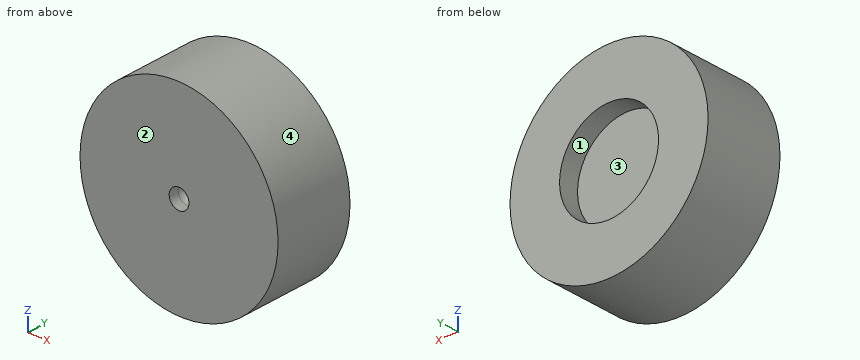
from build123d import *

# Parameters (mm, degrees)
SKETCH1_R           = 10
BOSS_EXTRUDE1_DEPTH = 8
SKETCH2_R           = 5
CUT_EXTRUDE1_DEPTH  = 2
SKETCH3_R           = 1
CUT_EXTRUDE2_DEPTH  = 2
FILLET1_R           = 1


with BuildPart() as part:
    # Sketch1 → Boss-Extrude1 (new body)
    with BuildSketch(Plane(origin=(0, 0, 0), x_dir=(1, 0, 0), z_dir=(0, 1, 0))):
        Circle(SKETCH1_R)
    extrude(amount=BOSS_EXTRUDE1_DEPTH)

    # Sketch2 → Cut-Extrude1 (cut)
    with BuildSketch(Plane(origin=(0, 8, 0), x_dir=(1, 0, 0), z_dir=(0, 1, 0))):
        Circle(SKETCH2_R)
    extrude(amount=-CUT_EXTRUDE1_DEPTH, mode=Mode.SUBTRACT)

    # Sketch3 → Cut-Extrude2 (cut)
    with BuildSketch(Plane.XZ):
        Circle(SKETCH3_R)
    extrude(amount=-CUT_EXTRUDE2_DEPTH, mode=Mode.SUBTRACT)

    # Fillet1
    fillet1_edges = [part.edges().sort_by_distance(p)[0] for p in [
        (-1, 2, 0),
    ]]
    fillet(fillet1_edges, radius=FILLET1_R)


solid = part.part
Read the model definition and answer for the solid it produces. Units are mm, in the model's axes. Face numbers are marked on the shaded views. Coordinates: 2 decimals unless noted, no trailing zeros. Loops run counter-clockwise (first coordinate to the right, second up) from the corner with the lowest first, then second, coordinate; pieces in that order, holes last. Notation, with made-up numbers: (85.5, 58) -> (106.5, 58) arc R15 ccw to (106.5, 72) -> close; hole circle Ø11 at (89.25, 34). An arc over 180 degrees is marked (long way). Answer in a Markdown table with one row per item.
Item 1: A cutting plane is placed at B-B on y = 0.75. Determine the outline of the cut face in (x, z).
Returned:
| item | result |
|---|---|
| outline | circle Ø20 at (0, 0); hole circle Ø2 at (0, 0) |
Item 2: A cutting plane is placed at C-C on z = 0. Determine the outline of the cut face in (x, y), plus the area to 3 significant figures.
Returned:
| item | result |
|---|---|
| outline | (-10, 0) -> (-1, 0) -> (-1, 1) arc R1 cw to (1, 1) -> (1, 0) -> (10, 0) -> (10, 8) -> (5, 8) -> (5, 6) -> (-5, 6) -> (-5, 8) -> (-10, 8) -> close |
| area | 136 mm^2 |
Item 3: For a pull along Z with two mould halves and no side action, classify the marked faces 1, 2, 3 and 4 as released by +Z, released by -Z, zero draft, split by the parting line, or undercut.
Returned:
| item | result |
|---|---|
| face 1 | undercut |
| face 2 | zero draft |
| face 3 | undercut |
| face 4 | split by the parting line |
Item 4: A cutting plane is placed at A-A on x = 0. Determine the outline of the cut face in (y, z).
Returned:
| item | result |
|---|---|
| outline | (0, -10) -> (8, -10) -> (8, -5) -> (6, -5) -> (6, 5) -> (8, 5) -> (8, 10) -> (0, 10) -> (0, 1) -> (1, 1) arc R1 cw to (1, -1) -> (0, -1) -> close |
Item 5: Straight lines are drawn through the part: line 1 along Z through (x, y) = (0, 7.4); line 2 along Z through (x, y) = (0, 0.2). For each, find the intervals that lie inside material, in ascending order. Write a range as [from, to].
Returned:
| item | result |
|---|---|
| line 1 | z = [-10, -5], [5, 10] |
| line 2 | z = [-10, -1], [1, 10] |
Item 6: A cutting plane is placed at D-D on x = -2.5. Determine the outline of the cut face in (y, z), plus the area to 3 significant figures.
Returned:
| item | result |
|---|---|
| outline | (0, -9.68) -> (8, -9.68) -> (8, -4.33) -> (6, -4.33) -> (6, 4.33) -> (8, 4.33) -> (8, 9.68) -> (0, 9.68) -> close |
| area | 138 mm^2 |
Item 7: Each of these flat-tipped pins is pushed along its axis until it touches: P1, Ø4, axis at y = 2.5, z = -4, coming from the +X side; P2, Ø3, axis at y = 3.5, z = 7, coming from the -X side; P3, Ø6, axis at x = 0, z = 0, coming from the +Y side. Where does it stop, or does it pass through?
Returned:
| item | result |
|---|---|
| P1 | stops at x = 9.8 |
| P2 | stops at x = -8.35 |
| P3 | stops at y = 6 |
